Build history of the part. All positions in model axes, mm. A direction names the side the tool comes from. Coordinates: 2 decimals unless noted, no trailing zeros. Write each loop counter-clockwise with the first axis right and the second up, starting at its lowest first coordinate (ties: lowest second). Pieces come first, ordered by that corner, then holes.
from build123d import *

# Parameters (mm, degrees)
SKETCH001_W  = 76
SKETCH001_H  = 76
SKETCH001_R  = 2
PAD_DEPTH    = 4
POCKET_DEPTH = 5
FILLET_R     = 10
CHAMFER_SIZE = 1


with BuildPart() as part:
    # Sketch001 → Pad (new body)
    with BuildSketch(Plane.XY):
        Rectangle(SKETCH001_W, SKETCH001_H)
        with Locations((-30.479838, 30.479838)):
            Circle(SKETCH001_R, mode=Mode.SUBTRACT)
        with Locations((30.479838, 30.479838)):
            Circle(SKETCH001_R, mode=Mode.SUBTRACT)
        with Locations((30.479838, -30.479838)):
            Circle(SKETCH001_R, mode=Mode.SUBTRACT)
        with Locations((-30.479838, -30.479838)):
            Circle(SKETCH001_R, mode=Mode.SUBTRACT)
        Circle(SKETCH001_R, mode=Mode.SUBTRACT)
    extrude(amount=PAD_DEPTH)

    # Sketch (on Face11 of Pad) → Pocket (cut)
    with BuildSketch(Plane.XY.offset(4)):
        Polygon((-29.826775, 20.627172), (-29.826775, -20.627172), (-22.363682, -28.4412), (-6.952969, -28.4412), (-6.952969, 28.4412), (-22.363682, 28.4412), align=None)
        Polygon((29.826775, 20.627172), (29.826775, -20.627172), (22.363682, -28.4412), (6.952969, -28.4412), (6.952969, 28.4412), (22.363682, 28.4412), align=None)
    extrude(amount=-POCKET_DEPTH, mode=Mode.SUBTRACT)

    # Fillet
    fillet_edges = [part.edges().sort_by_distance(p)[0] for p in [
        (38, -38, 2),
        (-38, -38, 2),
        (-38, 38, 2),
        (38, 38, 2),
    ]]
    fillet(fillet_edges, radius=FILLET_R)

    # Chamfer
    chamfer_edges = [part.edges().sort_by_distance(p)[0] for p in [
        (38, 0, 4),
        (35.071068, -35.071068, 4),
        (35.071068, 35.071068, 4),
        (0, -38, 4),
        (0, 38, 4),
        (-35.071068, -35.071068, 4),
        (-35.071068, 35.071068, 4),
        (-38, 0, 4),
        (-32.479838, -30.479838, 4),
        (28.479838, -30.479838, 4),
        (-29.826775, 0, 4),
        (-26.095228, -24.534186, 4),
        (-14.658325, -28.4412, 4),
        (-6.952969, 0, 4),
        (-14.658325, 28.4412, 4),
        (-26.095228, 24.534186, 4),
        (-32.479838, 30.479838, 4),
        (-2, 0, 4),
        (26.095228, 24.534186, 4),
        (14.658325, 28.4412, 4),
        (6.952969, 0, 4),
        (14.658325, -28.4412, 4),
        (26.095228, -24.534186, 4),
        (29.826775, 0, 4),
        (28.479838, 30.479838, 4),
        (38, 0, 0),
        (35.071068, -35.071068, 0),
        (35.071068, 35.071068, 0),
        (0, -38, 0),
        (0, 38, 0),
        (-35.071068, -35.071068, 0),
        (-35.071068, 35.071068, 0),
        (-38, 0, 0),
        (-32.479838, -30.479838, 0),
        (28.479838, -30.479838, 0),
        (-29.826775, 0, 0),
        (-26.095228, -24.534186, 0),
        (-14.658325, -28.4412, 0),
        (-6.952969, 0, 0),
        (-14.658325, 28.4412, 0),
        (-26.095228, 24.534186, 0),
        (-32.479838, 30.479838, 0),
        (-2, 0, 0),
        (26.095228, 24.534186, 0),
        (14.658325, 28.4412, 0),
        (6.952969, 0, 0),
        (14.658325, -28.4412, 0),
        (26.095228, -24.534186, 0),
        (29.826775, 0, 0),
        (28.479838, 30.479838, 0),
    ]]
    chamfer(chamfer_edges, length=CHAMFER_SIZE)


solid = part.part
(1) Two-plate mould, pull along X, no slides. Class faces 1 (the flat face through (26.386, 24.943, 0.507)), 2 (the conical face through (34.415, -34.558, 3.826)), 3 (the flat face through (6.953, 0, 2)), 4 (the cylindrical face through (-35.15, -34.99, 2.01)): pulls with the +X half, pulls with the -X half, needs draft (parallel to the pull), parting line crosses it, or undercut.
(2) 3-axis set-ups, long thin cutter, end or side, ignore diameter. For faces 5 (the flat face through (-29.827, 0, 2)), 6 (the conical face through (-34.558, -34.415, 3.826)), 7 (the flat face through (26.386, 24.943, 3.493)): which of +Z, -Z, +X, -X, +Y, -Y reach the whole face in a straight line?
(3) Slice it at D-D, the plane y = -25.5. List the corners of the cut face in (x, z), and give its area (3 significant figures).
(4) Probe L1, parallel to X at y = 20.5, z = 2.5; L2, parallel to Y at x = 0, z = 1.8; L3, parallel to X at y = -26, z = 3.3. List the from-to ranges inside material, lowest first.
(5) Slice it at A-A, the plane x = 19.5. List the corners of the cut face in (y, z).
(6) Slice it at B-B, the plane y = 0. Give the number of separate pieces and of enclosed holes in the cut face, and give its area (3 significant figures).
(7) Flat gauge pins, fed straight in: P1, Ø6.5, axis at x = 0, y = 0, coming from the +Z side; P2, Ø4.5, axis at x = -30.48, y = 30.48, coming from the -Z side. Where does each tip first touch, or does it go through?
(8) Slice it at C-C, the plane z = 2. List the corners of the cut face in (x, y).
Results:
1. face 1: undercut
1. face 2: pulls with the +X half
1. face 3: undercut
1. face 4: pulls with the -X half
2. face 5: +Z, -Z
2. face 6: +Z, -X, -Y
2. face 7: +Z
3. outline: (-38, 1) - (-37, 0) - (-26.56, 0) - (-25.17, 1) - (-25.17, 3) - (-26.56, 4) - (-37, 4) - (-38, 3) - close; (-6.95, 1) - (-5.95, 0) - (5.95, 0) - (6.95, 1) - (6.95, 3) - (5.95, 4) - (-5.95, 4) - (-6.95, 3) - close; (25.17, 1) - (26.56, 0) - (37, 0) - (38, 1) - (38, 3) - (37, 4) - (26.56, 4) - (25.17, 3) - close
3. area: 151 mm2
4. L1: x = -38 to -29.83, -6.95 to 6.95, 29.83 to 38
4. L2: y = -38 to -2, 2 to 38
4. L3: x = -37.7 to -25.11, -6.65 to 6.65, 25.11 to 37.7
5. outline: (-38, 1) - (-37, 0) - (-29.44, 0) - (-28.44, 1) - (-28.44, 3) - (-29.44, 4) - (-37, 4) - (-38, 3) - close; (28.44, 1) - (29.44, 0) - (37, 0) - (38, 1) - (38, 3) - (37, 4) - (29.44, 4) - (28.44, 3) - close
6. separate pieces: 4
6. enclosed holes: 0
6. area: 97.0 mm2
7. P1: stops at z = 4
7. P2: stops at z = 0.75
8. outline: (-38, -28) arc R10 ccw to (-28, -38) - (28, -38) arc R10 ccw to (38, -28) - (38, 28) arc R10 ccw to (28, 38) - (-28, 38) arc R10 ccw to (-38, 28) - close; hole circle Ø4 at (-30.48, -30.48); hole circle Ø4 at (-30.48, 30.48); hole (-29.83, -20.63) - (-22.36, -28.44) - (-6.95, -28.44) - (-6.95, 28.44) - (-22.36, 28.44) - (-29.83, 20.63) - close; hole circle Ø4 at (0, 0); hole (6.95, -28.44) - (22.36, -28.44) - (29.83, -20.63) - (29.83, 20.63) - (22.36, 28.44) - (6.95, 28.44) - close; hole circle Ø4 at (30.48, -30.48); hole circle Ø4 at (30.48, 30.48)
